Autodesk Inventor part; units mm, degrees
ref_plane "YZ Plane" through (0, 0, 0) normal (1, 0, 0) x (0, 1, 0)
ref_plane "XZ Plane" through (0, 0, 0) normal (0, 1, 0) x (-1, 0, 0)
ref_plane "XY Plane" through (0, 0, 0) normal (0, 0, 1) x (1, 0, 0)
sketch "Sketch1" plane through (0, 0, 0) normal (0, 0, 1) x (1, 0, 0)
  circle A0 centre (-12, 9) radius 6
  circle A1 centre (-12, -9) radius 6
  circle A2 centre (-28, 23) radius 2
  circle A3 centre (-28, -23) radius 2
  arc A4 (-31.4115, -18.0643) -> (-23.8208, -27.3051) centre (-28, -23) ccw
  arc A5 (-23.8208, 27.3051) -> (-31.4115, 18.0643) centre (-28, 23) ccw
  line L0 (-28, 23) -> (-28, -23) construction
  circle A6 centre (0, 0) radius 36.2353 construction
  arc A7 (-11.7365, -34.282) -> (0.0617, -36.2353) centre (-5.9186, -35.7487) ccw
  circle A8 centre (-5.9186, -35.7487) radius 2
  arc A9 (31.3499, -18.171) -> (35.5573, -6.9768) centre (33.9186, -12.7487) ccw
  circle A10 centre (33.9186, -12.7487) radius 2
  arc A11 (35.5573, 6.9768) -> (31.3499, 18.171) centre (33.9186, 12.7487) ccw
  circle A12 centre (33.9186, 12.7487) radius 2
  arc A13 (0.0617, 36.2353) -> (-11.7365, 34.282) centre (-5.9186, 35.7487) ccw
  circle A14 centre (-5.9186, 35.7487) radius 2
  line L1 (33.9186, 12.7487) -> (33.9186, -12.7487) construction
  line L2 (-34, 23) -> (-34, -23)
  line L3 (39.9186, 12.7487) -> (39.9186, -12.7487)
  line L4 (-31, 28.1962) -> (-8.9186, 40.9449)
  line L5 (-2.9186, 40.9449) -> (36.9186, 17.9449)
  line L6 (36.9186, -17.9449) -> (-2.9186, -40.9449)
  line L7 (-31, -28.1962) -> (-8.9186, -40.9449)
  dimension "d0" = 12
  dimension "d1" = 12
  dimension "d4" = 4
  dimension "d5" = 4
  dimension "d6" = 46
  dimension "d7" = 23
  dimension "d8" = 28
  dimension "d9" = 28
  dimension "d10" = 12
  dimension "d11" = 12
  dimension "d15" = 360
  dimension "d42" = 25.4974
  dimension "d45" = 9
  dimension "d46" = 9
  dimension "d48" = 22
  dimension "d49" = 22
extrude "Extrusion1" add sketch "Sketch1" along normal blind 5
sketch "Sketch2" plane through (0, 0, 5) normal (0, 0, 1) x (1, 0, 0)
  circle A0 centre (-12, 9) radius 6
  circle A1 centre (-12, -9) radius 6
  circle A2 centre (-9, 0) radius 1.5
  circle A3 centre (-21, 8.5) radius 1.5
  circle A4 centre (-21, -8.5) radius 1.5
  point P0 (0, 0)
  dimension "d19" = 3
  dimension "d20" = 3
  dimension "d21" = 3
  dimension "d23" = 21
  dimension "d24" = 21
  dimension "d25" = 17
  dimension "d26" = 8.5
  dimension "d47" = 9
extrude "Extrusion2" cut sketch "Sketch2" against normal through all contours A2 | A3 | A4
sketch "Sketch3" plane through (0, 0, 5) normal (0, 0, 1) x (1, 0, 0)
  circle A0 centre (14.9186, 14) radius 1.5
  circle A1 centre (14.9186, -14) radius 1.5
  line L0 (39.9186, -12.7487) -> (39.9186, 12.7487)
  point P0 (0, 0)
  dimension "d29" = 3
  dimension "d30" = 3
  dimension "d31" = 28
  dimension "d33" = 14
  dimension "d77" = 25
  dimension "d78" = 25
extrude "Extrusion3" cut sketch "Sketch3" against normal through all
sketch "Sketch6" plane through (0, 0, 5) normal (0, 0, 1) x (1, 0, 0)
  arc A0 (22.75, -18) -> (24.75, -16) centre (22.75, -16) ccw
  line L0 (22.75, -18) -> (17.25, -18)
  arc A1 (15.25, -16) -> (17.25, -18) centre (17.25, -16) ccw
  line L1 (15.25, -16) -> (15.25, 16)
  arc A2 (17.25, 18) -> (15.25, 16) centre (17.25, 16) ccw
  line L2 (17.25, 18) -> (22.75, 18)
  arc A3 (24.75, 16) -> (22.75, 18) centre (22.75, 16) ccw
  line L3 (24.75, 16) -> (24.75, -16)
  circle A4 centre (20, -14) radius 1.5
  circle A5 centre (20, 14) radius 1.5
  circle A6 centre (21.75, -3) radius 1
  point P0 (0, 0)
extrude "Extrusion5" cut sketch "Sketch6" against normal through all contours A6
thread "Thread1"
thread "Thread2"
thread "Thread3"
thread "Thread4"
thread "Thread5"
thread "Thread6"
sketch "Sketch8" plane through (0, 0, 5) normal (0, 0, 1) x (1, 0, 0)
  circle A0 centre (-28, 23) radius 2
  circle A1 centre (-5.9186, 35.7487) radius 2
  circle A2 centre (33.9186, 12.7487) radius 2
  circle A3 centre (33.9186, -12.7487) radius 2
  circle A4 centre (-5.9186, -35.7487) radius 2
  circle A5 centre (-28, -23) radius 2
  circle A6 centre (21.75, -3) radius 1
  circle A7 centre (14.9186, 14) radius 1.5
  circle A8 centre (14.9186, -14) radius 1.5
  circle A9 centre (-21, 8.5) radius 1.5
  circle A10 centre (-9, 0) radius 1.5
  circle A11 centre (-21, -8.5) radius 1.5
  circle A12 centre (-12, -9) radius 6
  circle A13 centre (-12, 9) radius 6
  circle A14 centre (-5.9186, 35.7487) radius 2
  circle A15 centre (33.9186, 12.7487) radius 2
  circle A16 centre (33.9186, -12.7487) radius 2
  circle A17 centre (-5.9186, -35.7487) radius 2
  circle A18 centre (-28, -23) radius 2
  circle A19 centre (-28, 23) radius 2
  arc A20 (-31, 28.1962) -> (-34, 23) centre (-28, 23) ccw
  line L0 (-34, 23) -> (-34, -23)
  arc A21 (-34, -23) -> (-31, -28.1962) centre (-28, -23) ccw
  line L1 (-31, -28.1962) -> (-8.9186, -40.9449)
  arc A22 (-8.9186, -40.9449) -> (-2.9186, -40.9449) centre (-5.9186, -35.7487) ccw
  line L2 (-2.9186, -40.9449) -> (36.9186, -17.9449)
  arc A23 (36.9186, -17.9449) -> (39.9186, -12.7487) centre (33.9186, -12.7487) ccw
  line L3 (39.9186, -12.7487) -> (39.9186, 12.7487)
  arc A24 (39.9186, 12.7487) -> (36.9186, 17.9449) centre (33.9186, 12.7487) ccw
  line L4 (36.9186, 17.9449) -> (-2.9186, 40.9449)
  arc A25 (-2.9186, 40.9449) -> (-8.9186, 40.9449) centre (-5.9186, 35.7487) ccw
  line L5 (-8.9186, 40.9449) -> (-31, 28.1962)
  circle A26 centre (-28, 23) radius 3.5
  circle A27 centre (-5.9186, 35.7487) radius 3.5
  circle A28 centre (33.9186, 12.7487) radius 3.5
  circle A29 centre (33.9186, -12.7487) radius 3.5
  circle A30 centre (-5.9186, -35.7487) radius 3.5
  circle A31 centre (-28, -23) radius 3.5
  point P0 (0, 0)
  dimension "d62" = 1.5
  dimension "d63" = 1.5
  dimension "d64" = 1.5
  dimension "d65" = 1.5
  dimension "d66" = 1.5
  dimension "d67" = 1.5
extrude "Extrusion6" cut sketch "Sketch8" against normal blind 2 contours L5 A25 L4 A24 L3 A23 L2 A22 L1 A21 L0 A20
sketch "Sketch9" plane through (-28, -23, 5) normal (0, 0, 1) x (1, 0, 0)
  circle A0 centre (0, 0) radius 3.5
  circle A1 centre (0, 46) radius 3.5
  circle A2 centre (22.0814, 58.7487) radius 2
  circle A3 centre (22.0814, 58.7487) radius 3.5
  circle A4 centre (0, 46) radius 2
  circle A5 centre (0, 0) radius 2
  circle A6 centre (22.0814, -12.7487) radius 3.5
  circle A7 centre (22.0814, -12.7487) radius 2
  circle A8 centre (61.9186, 10.2513) radius 3.5
  circle A9 centre (61.9186, 10.2513) radius 2
  circle A10 centre (61.9186, 35.7487) radius 2
  circle A11 centre (61.9186, 35.7487) radius 3.5
  point P0 (28, 23)
extrude "Extrusion7" add sketch "Sketch9" along normal blind 2
sketch "Sketch10" plane through (0, 0, 3) normal (0, 0, 1) x (1, 0, 0)
  circle A0 centre (-12, 9) radius 6
  circle A1 centre (-12, -9) radius 6
  circle A2 centre (-28, -23) radius 3.5
  circle A3 centre (-5.9186, -35.7487) radius 3.5
  circle A4 centre (33.9186, -12.7487) radius 3.5
  circle A5 centre (33.9186, 12.7487) radius 3.5
  circle A6 centre (-5.9186, 35.7487) radius 3.5
  circle A7 centre (-28, 23) radius 3.5
  circle A8 centre (-21, -8.5) radius 1.5
  circle A9 centre (-9, 0) radius 1.5
  circle A10 centre (-21, 8.5) radius 1.5
  circle A11 centre (14.9186, -14) radius 1.5
  circle A12 centre (14.9186, 14) radius 1.5
  circle A13 centre (21.75, -3) radius 1
  arc A14 (-31, 28.1962) -> (-34, 23) centre (-28, 23) ccw
  line L0 (-34, -23) -> (-34, 23)
  arc A15 (-34, -23) -> (-31, -28.1962) centre (-28, -23) ccw
  line L1 (-8.9186, -40.9449) -> (-31, -28.1962)
  arc A16 (-8.9186, -40.9449) -> (-2.9186, -40.9449) centre (-5.9186, -35.7487) ccw
  line L2 (36.9186, -17.9449) -> (-2.9186, -40.9449)
  arc A17 (36.9186, -17.9449) -> (39.9186, -12.7487) centre (33.9186, -12.7487) ccw
  line L3 (39.9186, 12.7487) -> (39.9186, -12.7487)
  arc A18 (39.9186, 12.7487) -> (36.9186, 17.9449) centre (33.9186, 12.7487) ccw
  line L4 (-2.9186, 40.9449) -> (36.9186, 17.9449)
  arc A19 (-2.9186, 40.9449) -> (-8.9186, 40.9449) centre (-5.9186, 35.7487) ccw
  line L5 (-31, 28.1962) -> (-8.9186, 40.9449)
  arc A20 (-32, 29.9282) -> (-36, 23) centre (-28, 23) ccw
  line L6 (-32, 29.9282) -> (-9.9186, 42.6769)
  arc A21 (-1.9186, 42.6769) -> (-9.9186, 42.6769) centre (-5.9186, 35.7487) ccw
  line L7 (-1.9186, 42.6769) -> (37.9186, 19.6769)
  arc A22 (41.9186, 12.7487) -> (37.9186, 19.6769) centre (33.9186, 12.7487) ccw
  line L8 (41.9186, 12.7487) -> (41.9186, -12.7487)
  arc A23 (37.9186, -19.6769) -> (41.9186, -12.7487) centre (33.9186, -12.7487) ccw
  line L9 (37.9186, -19.6769) -> (-1.9186, -42.6769)
  arc A24 (-9.9186, -42.6769) -> (-1.9186, -42.6769) centre (-5.9186, -35.7487) ccw
  line L10 (-9.9186, -42.6769) -> (-32, -29.9282)
  arc A25 (-36, -23) -> (-32, -29.9282) centre (-28, -23) ccw
  line L11 (-36, -23) -> (-36, 23)
  point P0 (0, 0)
  dimension "d72" = 2
extrude "Extrusion8" add sketch "Sketch10" against normal up to surface (3 mm away) contours L6 A21 L7 A22 L8 A23 L9 A24 L10 A25 L11 A20
sketch "Sketch11" plane through (0, 0, 0) normal (0, 0, -1) x (-1, 0, 0)
  circle A0 centre (-33.4186, 0) radius 1.5
  line L0 (-41.9186, 12.7487) -> (-41.9186, -12.7487)
  line L1 (0, 0) -> (-49.8844, 0) construction
  circle A1 centre (16.7093, -28.9413) radius 1.5
  circle A2 centre (16.7093, 28.9413) radius 1.5
  dimension "d97" = 8.5
  dimension "d98" = 0
  dimension "d101" = 360
extrude "Extrusion9" cut sketch "Sketch11" against normal through all
sketch "Sketch12" plane through (0, 0, 3) normal (0, 0, 1) x (1, 0, 0)
  arc A0 (12.7181, 3.8928) -> (13.6045, 2.1) centre (13.1686, 3) ccw
  circle A1 centre (13.1686, 3) radius 1
  point P0 (0, 0)
extrude "Extrusion10" cut sketch "Sketch12" against normal through all
sketch "Sketch13" plane through (0, 0, 0) normal (0, 0, -1) x (-1, 0, 0)
  line L0 (6, 15) -> (6, -15)
  line L1 (24, 15) -> (6, 15)
  line L2 (24, -15) -> (6, -15)
  line L3 (9.9186, -42.6769) -> (32, -29.9282)
  line L4 (3.1479, -25) -> (18.1479, -25)
  line L5 (18.1479, -25) -> (18.1479, -17)
  line L6 (18.1479, -17) -> (3.1479, -17)
  line L7 (3.1479, -17) -> (3.1479, -25)
  point P0 (0, 0)
  dimension "d84" = 8
  dimension "d85" = 15
  dimension "d86" = 2
extrude "Extrusion11" cut sketch "Sketch13" against normal through all
mirror "Mirror1" about plane through (0, 0, 0) normal (0, 1, 0) of "Extrusion11"
sketch "Sketch14" plane through (0, 0, 3) normal (0, 0, 1) x (1, 0, 0)
  circle A0 centre (-27.5, 0) radius 1.5
  line L0 (-36, -23) -> (-36, 23)
  circle A1 centre (13.75, -23.8157) radius 1.5
  circle A2 centre (13.75, 23.8157) radius 1.5
  point P0 (0, 0)
  dimension "d89" = 3
  dimension "d90" = 8.5
  dimension "d93" = 360
extrude "Extrusion12" cut sketch "Sketch14" against normal through all
equation "\"d1\" = d0"
equation "\"d5\" = d4"
equation "\"d10\" = d11"
equation "\"d49\" = d48"
equation "\"d78\" = d77"
properties part number "efector"
Geometry check sheet. Reference: the model listing, model coordinates, mm. A direction names the side the tool comes from. Coordinates: 2 decimals unless noted, no trailing zeros. Order: outer loops, then holes, each group sorted by start corner. A loop starts at its lowest first (then second) coordinate and runs counter-clockwise, first axis right, second up. Notation, with made-up numbers: (1.5, 60.25) - (56.5, 60.25) arc R27 cw to (56.5, 78.25) - close; hole circle Ø9 at (81, 53.5). An arc over 180 degrees is marked (long way). Answer in a Markdown table with one row per item. Add a question column.
1. Section check A-A (y = 0). Enter the section's corners in (x, z), plus the area to 3 significant figures.
2. Draft check along X on faces 4 (the face through (34, -15, 7)), 5 (the face through (-26.12, 25.95, 5.03)), 6 (the face through (34.61, -0.91, 1.48)). Enter one of: +X half, -X half, draft (parallel to the pull), parting line (faces both ways), or undercut.
3. Material ranges on L1, parallel to Y at x = -12, z = 2.3; L2, parallel to Y at x = -14, z = 2; L3, parallel to Y at x = -28, z = 2.5, recorded low to high. Write a range as [from, to].
4. Section check C-C (z = 4). Give the number of separate pieces and of enclosed holes in the cut face, plus the area to 3 significant figures.
5. Access from +Z, -Z, +X, -X, +Y, -Y to the whole of each face (thin tool, end or side, straight path). Record for faces 1 (the face through (-34.957, -26.949, 1.521)), 2 (the face through (2, 1, 3)), 3 (the face through (-11, -25, 1)).
6. Section check B-B (x = -27.5). Enter the section's corners in (y, z).
7. Gauge pin test, flat ends, axial feed: pin 1 Ø0.9 at (x, z) = (-9.5, 1) entering from +Y; pin 2 Ø1.5 at (y, z) = (24, 4) entering from -X; pin 3 Ø10 at (x, y) = (-10.5, -3.5) entering from +Z; pin 4 Ø3 at (x, y) = (-28, 23) entering from +Z. Record the tip position at first contact, or that the pin passes through.
8. Section check D-D (x = -5). Enter the section's corners in (y, z), plus the area to 3 significant figures.
Data:
| question | item | result |
|---|---|---|
| 1 | outline | (-36, 0) - (-29, 0) - (-29, 3) - (-36, 3) - close; (-26, 0) - (-10.5, 0) - (-10.5, 3) - (-26, 3) - close; (-7.5, 0) - (31.92, 0) - (31.92, 3) - (-7.5, 3) - close; (34.92, 0) - (41.92, 0) - (41.92, 3) - (34.92, 3) - close |
| 1 | area | 207 mm² |
| 2 | face 4 | draft |
| 2 | face 5 | parting line |
| 2 | face 6 | undercut |
| 3 | L1 | y = [-41.48, -25], [-17, -15], [-3, 3], [15, 17], [25, 41.48] |
| 3 | L2 | y = [-40.32, -25], [-17, -14.66], [-3.34, 3.34], [14.66, 17], [25, 40.32] |
| 3 | L3 | y = [-32.24, -25], [-21, -1.41], [1.41, 21], [25, 32.24] |
| 4 | separate pieces | 6 |
| 4 | enclosed holes | 6 |
| 4 | area | 156 mm² |
| 5 | face 1 | +Z, -Z, -X, -Y |
| 5 | face 2 | +Z |
| 5 | face 3 | +Z, -Z |
| 6 | outline | (-32.53, 0) - (-24.94, 0) - (-24.94, 7) - (-26.46, 7) - (-26.46, 3) - (-32.53, 3) - close; (-21.06, 0) - (-1.5, 0) - (-1.5, 3) - (-19.54, 3) - (-19.54, 7) - (-21.06, 7) - close; (1.5, 0) - (21.06, 0) - (21.06, 7) - (19.54, 7) - (19.54, 3) - (1.5, 3) - close; (24.94, 0) - (32.53, 0) - (32.53, 3) - (26.46, 3) - (26.46, 7) - (24.94, 7) - close |
| 7 | pin 1 | stops at y = 43.11 |
| 7 | pin 2 | stops at x = -31.49 |
| 7 | pin 3 | stops at z = 3 |
| 7 | pin 4 | passes through |
| 8 | outline | (-43.7, 0) - (-37.53, 0) - (-37.53, 7) - (-39.13, 7) - (-39.13, 3) - (-43.7, 3) - close; (-33.97, 0) - (-25, 0) - (-25, 3) - (-32.37, 3) - (-32.37, 7) - (-33.97, 7) - close; (-17, 0) - (17, 0) - (17, 3) - (-17, 3) - close; (25, 0) - (33.97, 0) - (33.97, 7) - (32.37, 7) - (32.37, 3) - (25, 3) - close; (37.53, 0) - (43.7, 0) - (43.7, 3) - (39.13, 3) - (39.13, 7) - (37.53, 7) - close |
| 8 | area | 218 mm² |
